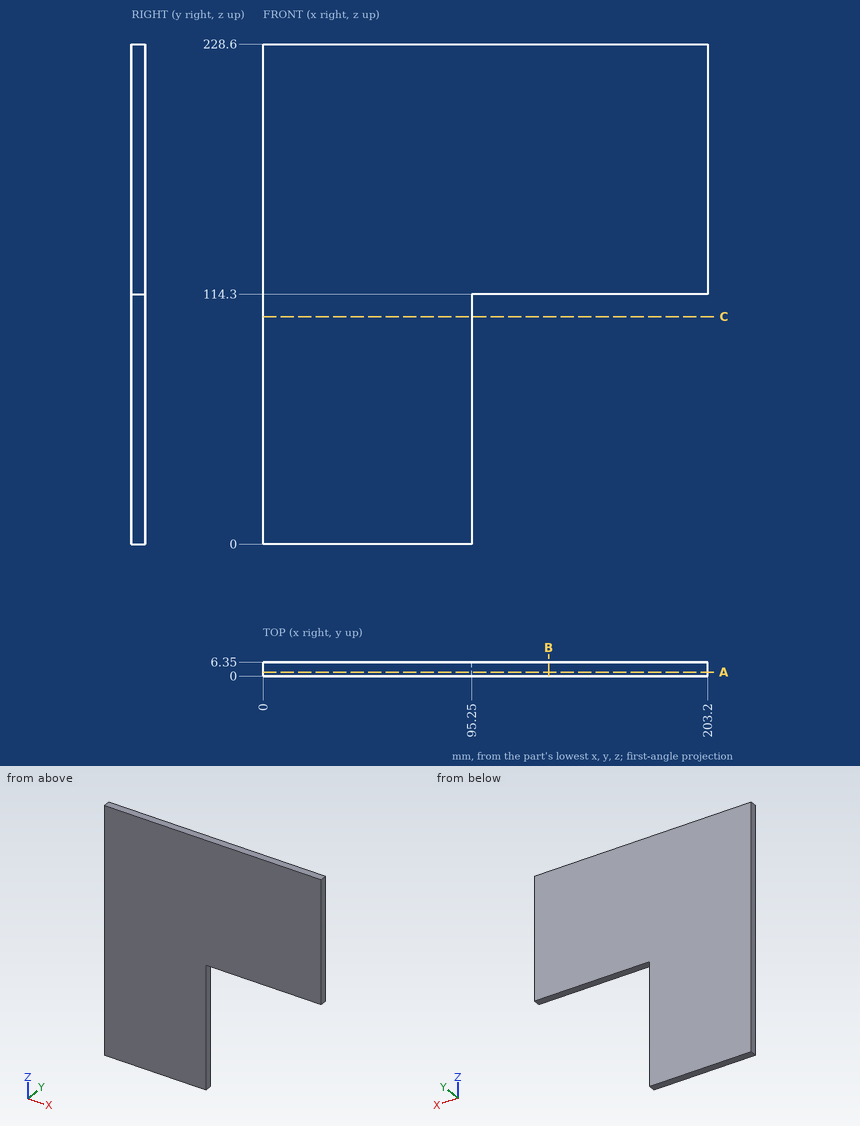
The drawing under review shows one solid part. Ordinate dimensions are in mm from its lowest x, y, z. Coordinates: 2 decimals unless noted, no trailing zeros. Loops run counter-clockwise (first coordinate to the right, second up) from the corner with the lowest first, then second, coordinate; pieces in that order, holes last. Notation, with made-up numbers: (-20.5, 59.25) - (28.5, 59.25) arc R14 cw to (28.5, 81.25) - close; hole circle Ø11 at (7.25, 74). An arc over 180 degrees is marked (long way). Return JSON: item names as keys, results as strings.
Item 1: Insertion check: pin 1 (1.5 mm diameter, centred on y = 0.5, z = 24, fed in from +X). The pin has a flat end and moves straight along its axis. Give the tip position at first contact, or say it passes through.
Determined:
{"pin 1": "stops at x = 95.25"}
Item 2: Take a section at C-C (z = 104). Give the boundary of the cut face in (x, y), then the cut area to 3 significant figures.
Determined:
{"outline": "(0, 0) - (95.25, 0) - (95.25, 6.35) - (0, 6.35) - close", "area": "605 mm2"}
Item 3: For line 1 (X direction, y = 2.25, z = 54); line 2 (Z direction, x = 144.5, y = 1), list the stretches that pass through material, from the lowest coordinate up.
Determined:
{"line 1": "x = 0 to 95.25", "line 2": "z = 114.3 to 228.6"}
Item 4: Take a section at A-A (y = 1.75). Give the boundary of the cut face in (x, z).
Determined:
{"outline": "(0, 0) - (95.25, 0) - (95.25, 114.3) - (203.2, 114.3) - (203.2, 228.6) - (0, 228.6) - close"}
Item 5: Take a section at B-B (x = 130.5). Give the boundary of the cut face in (y, z), then the cut area to 3 significant figures.
Determined:
{"outline": "(0, 114.3) - (6.35, 114.3) - (6.35, 228.6) - (0, 228.6) - close", "area": "726 mm2"}
